```python
from build123d import *

# Parameters (mm, degrees)
SKETCH1_R           = 8.5
BOSS_EXTRUDE1_DEPTH = 2
SKETCH2_W           = 6.948756548
SKETCH2_H           = 6.57893477
BOSS_EXTRUDE2_DEPTH = 8
SKETCH3_R           = 1.5
CUT_EXTRUDE1_DEPTH  = 8
SKETCH1_2_R         = 8.5
BOSS_EXTRUDE3_DEPTH = 15
SKETCH5_R           = 7
CUT_EXTRUDE2_DEPTH  = 15


with BuildPart() as part:
    # Sketch1 → Boss-Extrude1 (new body)
    with BuildSketch(Plane(origin=(0, 0, 0), x_dir=(1, 0, 0), z_dir=(0, 1, 0))):
        Circle(SKETCH1_R)
    extrude(amount=BOSS_EXTRUDE1_DEPTH)

    # Sketch2 → Boss-Extrude2 (add)
    with BuildSketch(Plane(origin=(0, 2, 0), x_dir=(1, 0, 0), z_dir=(0, 1, 0))):
        Rectangle(SKETCH2_W, SKETCH2_H)
    extrude(amount=BOSS_EXTRUDE2_DEPTH)

    # Sketch3 → Cut-Extrude1 (cut)
    with BuildSketch(Plane.XY.offset(3.289467385)):
        with Locations((0, 6.248369683)):
            Circle(SKETCH3_R)
    extrude(amount=-CUT_EXTRUDE1_DEPTH, mode=Mode.SUBTRACT)

    # Sketch1_2 → Boss-Extrude3 (add)
    with BuildSketch(Plane(origin=(0, 0, 0), x_dir=(1, 0, 0), z_dir=(0, 1, 0))):
        Circle(SKETCH1_2_R)
    extrude(amount=-BOSS_EXTRUDE3_DEPTH)

    # Sketch5 → Cut-Extrude2 (cut)
    with BuildSketch(Plane(origin=(0, -15, 0), x_dir=(-1, 0, 0), z_dir=(0, -1, 0))):
        Circle(SKETCH5_R)
    extrude(amount=-CUT_EXTRUDE2_DEPTH, mode=Mode.SUBTRACT)


solid = part.part
```
The listing builds one solid part. Answer for the finished solid, in the listing's coordinates (mm). A direction names the side the tool comes from. Round coordinates to 2 decimals unless told otherwise and drop trailing zeros. Loops run counter-clockwise (first coordinate to the right, second up) from the corner with the lowest first, then second, coordinate; pieces in that order, holes last.
Q1. Which of the six approach directions +Z, -Z, +X, -X, +Y, -Y give full straight-line access (tool end or side, diameter ignored) to faces 4 (the face through (3.474, 6, 0)), 5 (the face through (0, 10, 0)), 6 (the face through (-2, 6, -3.289)), 7 (the face through (-2, 6, 3.289)), 8 (the face through (0, 0, 0))?
Q2. Section A-A, the plane x = 0 is taken. Determine the outline of the cut face in (y, z), then the cut area to 3 significant figures.
Q3. For a pull along X with two mould halves and no side action, classify faces 1 (the face through (-3.474, 6, 0)), 2 (the face through (-0.325, 4.784, 0.046)), 3 (the face through (4, 2, 0)) as released by +X, released by -X, zero draft, split by the parting line, or undercut.
Q4. Section D-D, the plane z = -6.25 is taken. Determine the outline of the cut face in (x, y).
Q5. Find the intervals of material crossed by line 1 (X direction, y = -8, z = 0); line 2 (Y direction, x = 0, z = 1.75), in increasing order.
Q6. Given pin 1 Ø4 at (y, z) = (-1.5, 0.5) entering from +X; pin 2 Ø2 at (y, z) = (7, 6) entering from -X; pin 3 Ø2 at (x, y) = (-1, 6.5) entering from +Z; pin 4 Ø2 at (x, z) = (4, -6.5) entering from +Y, each flat-ended and moving along its own axis, determine where each tip first touches the part or whether it passes through.
Q7. Section B-B, the plane z = 0 is taken. Determine the outline of the cut face in (x, y), then the cut area to 3 significant figures.
Q8. Section C-C, the plane y = 7.25 is taken. Determine the outline of the cut face in (x, z).
Completed:
1. face 4: +Z, -Z, +X, +Y
1. face 5: +Z, -Z, +X, -X, +Y
1. face 6: -Z, +X, -X, +Y
1. face 7: +Z, +X, -X, +Y
1. face 8: -Y
2. outline: (-15, -8.5) - (2, -8.5) - (2, -3.29) - (4.75, -3.29) - (4.75, 3.29) - (2, 3.29) - (2, 8.5) - (-15, 8.5) - (-15, 7) - (0, 7) - (0, -7) - (-15, -7) - close; (7.75, -3.29) - (10, -3.29) - (10, 3.29) - (7.75, 3.29) - close
2. area: 112 mm2
3. face 1: released by -X
3. face 2: undercut
3. face 3: zero draft
4. outline: (-5.76, -15) - (-3.15, -15) - (-3.15, 0) - (3.15, 0) - (3.15, -15) - (5.76, -15) - (5.76, 2) - (-5.76, 2) - close
5. line 1: x = -8.5 to -7, 7 to 8.5
5. line 2: y = 0 to 4.75, 7.75 to 10
6. pin 1: stops at x = 8.5
6. pin 2: passes through
6. pin 3: stops at z = 3.29
6. pin 4: stops at y = 2
7. outline: (-8.5, -15) - (-7, -15) - (-7, 0) - (7, 0) - (7, -15) - (8.5, -15) - (8.5, 2) - (3.47, 2) - (3.47, 10) - (-3.47, 10) - (-3.47, 2) - (-8.5, 2) - close; hole circle Ø3 at (0, 6.25)
7. area: 128 mm2
8. outline: (-3.47, -3.29) - (-1.12, -3.29) - (-1.12, 3.29) - (-3.47, 3.29) - close; (1.12, -3.29) - (3.47, -3.29) - (3.47, 3.29) - (1.12, 3.29) - close
